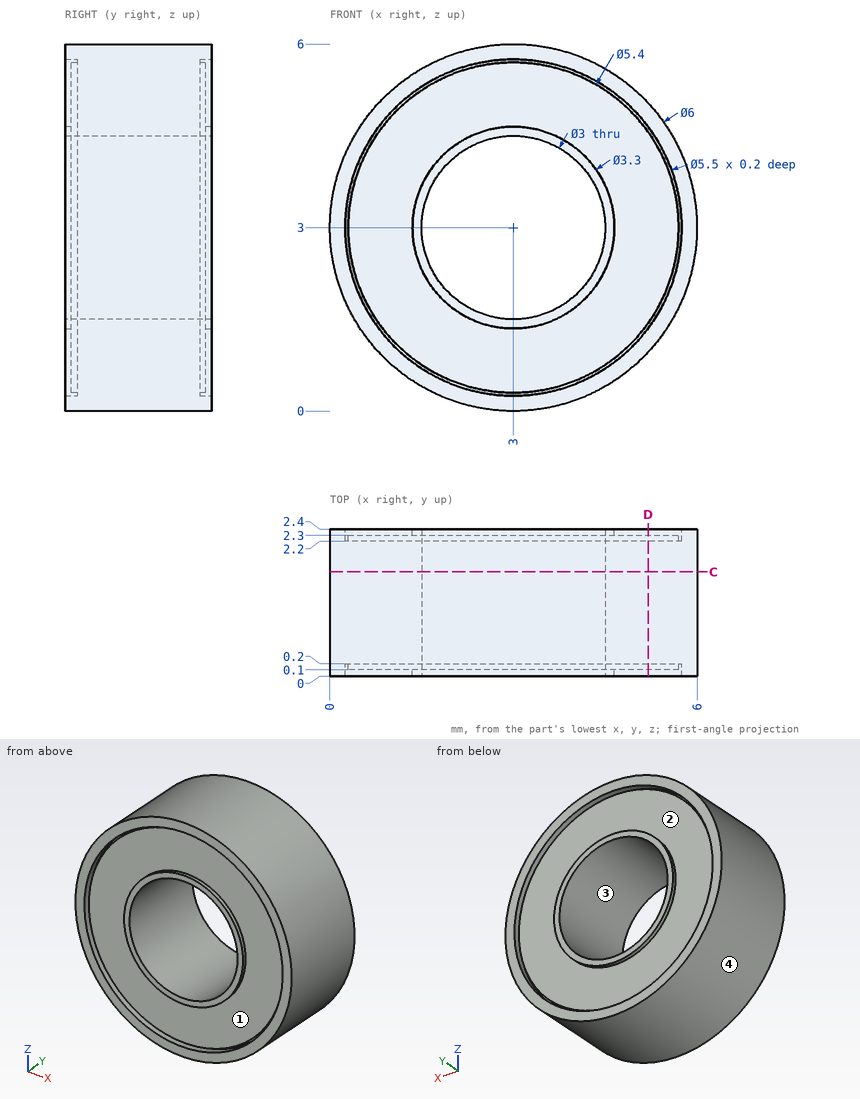
Here's the drawing with two shaded views (mm, measured from the low corner). I have some questions. A direction names the side the tool comes from. Coordinates: 2 decimals unless noted, no trailing zeros. Order: outer loops, then holes, each group sorted by start corner. A loop starts at its lowest first (then second) coordinate and runs counter-clockwise, first axis right, second up.
Item 1: I need wall thicknesses on probe 1 along Z at (x, y) = (3.5, 1); probe 2 along Y at (x, z) = (4.65, 4.9); probe 3 along Z at (x, y) = (2.7, 1.95). Which ranges of each line are inside material? Lowest first, please.
Response values:
probe 1: z = 0.04 to 1.59, 4.41 to 5.96
probe 2: y = 0.1 to 2.3
probe 3: z = 0.02 to 1.53, 4.47 to 5.98
Item 2: If we section it at D-D, the plane x = 5.2: List the corners of the cut face in (y, z) for me.
Response values:
outline: (0, 0.96) - (2.4, 0.96) - (2.4, 1.35) - (2.2, 1.35) - (2.2, 1.43) - (2.3, 1.43) - (2.3, 4.57) - (2.2, 4.57) - (2.2, 4.65) - (2.4, 4.65) - (2.4, 5.04) - (0, 5.04) - (0, 4.65) - (0.2, 4.65) - (0.2, 4.57) - (0.1, 4.57) - (0.1, 1.43) - (0.2, 1.43) - (0.2, 1.35) - (0, 1.35) - close
Item 3: I'm going to push a flat-ended pin straight in: pin 1 Ø2.5 at (x, z) = (4, 2.5) entering from +Y. Where does the tip first touch, or does it pass through?
Response values:
pin 1: stops at y = 2.4
Item 4: Thinking about a two-plate mould opening in Z: for the marked faces 3 and 4, which applies, pulls with the +Z half, pulls with the -Z half, needs draft (parallel to the pull), parting line crosses it, or undercut?
Response values:
face 3: undercut
face 4: parting line crosses it
Item 5: If we section it at C-C, the plane y = 1.7: List the corners of the cut face in (x, z) for me, then the cut area to 3 significant figures.
Response values:
outline: circle Ø6 at (3, 3); hole circle Ø3 at (3, 3)
area: 21.2 mm2
Item 6: Which directions (+Z, -Z, +X, -X, +Y, -Y) give clear straight access to the entire face, cutting with the end or side of a thin tool? Please do the marked faces 1 and 2.
Response values:
face 1: -Y
face 2: +Y
